from build123d import *

# Parameters (mm, degrees)
SKETCH1_W           = 76.2
SKETCH1_H           = 50.8
SKETCH1_R           = 3.175
SKETCH1_R_2         = 2.38125
BOSS_EXTRUDE1_DEPTH = 6.35


with BuildPart() as part:
    # Sketch1 → Boss-Extrude1 (new body)
    # profile 1 of 2: a face of its own
    with BuildSketch(Plane(origin=(0, 0, 0), x_dir=(1, 0, 0), z_dir=(0, 1, 0))):
        Rectangle(SKETCH1_W, SKETCH1_H)
        with Locations((25.4, 0)):
            Circle(SKETCH1_R, mode=Mode.SUBTRACT)
        with Locations(Location((-31.75, 0, 0), (0, 0, 270))):
            Circle(SKETCH1_R_2, mode=Mode.SUBTRACT)
    # profile 2 of 2: a face of its own
    with BuildSketch(Plane(origin=(0, 0, 0), x_dir=(1, 0, 0), z_dir=(0, 1, 0))):
        with Locations((25.4, 0)):
            Circle(SKETCH1_R)
    extrude(amount=BOSS_EXTRUDE1_DEPTH)


solid = part.part
Design review of the part built by this model. Coordinates are the model's own, in mm. Coordinates: 2 decimals unless noted, no trailing zeros. Order: outer loops, then holes, each group sorted by start corner. A loop starts at its lowest first (then second) coordinate and runs counter-clockwise, first axis right, second up.
Item 1: Take a section at B-B, the plane x = -31.75. Write out the cut boundary in (y, z), then the cut area to 3 significant figures.
Item 2: The part is to be moulded in two halves that separate along X. For faces 1 (the flat face through (-1, 0, 0)), 2 (the flat face through (-38.1, 3, 0)), 3 (the flat face through (38.1, 3, 0)), 4 (the cylindrical face through (-29.39, 3.13, -0.31)), say which applies: pulls with the +X half, pulls with the -X half, needs draft (parallel to the pull), parting line crosses it, or undercut.
Item 3: For pin 1 Ø1 at (x, z) = (8, -1) entering from -Y; pin 2 Ø3 at (x, z) = (-31.75, 0) entering from +Y, all flat-tipped, find the tip position at first contact; note any pin that passes through.
Item 4: Take a section at A-A, the plane z = 0. Write out the cut boundary in (x, y), then the cut area to 3 significant figures.
Item 5: For line 1 (X direction, y = 5, z = 0), list the stretches that pass through material, from the lowest coordinate up.
The answers:
1. outline: (0, -25.4) - (6.35, -25.4) - (6.35, -2.38) - (0, -2.38) - close; (0, 2.38) - (6.35, 2.38) - (6.35, 25.4) - (0, 25.4) - close
1. area: 292 mm2
2. face 1: needs draft
2. face 2: pulls with the -X half
2. face 3: pulls with the +X half
2. face 4: undercut
3. pin 1: stops at y = 0
3. pin 2: passes through
4. outline: (-38.1, 0) - (-34.13, 0) - (-34.13, 6.35) - (-38.1, 6.35) - close; (-29.37, 0) - (38.1, 0) - (38.1, 6.35) - (-29.37, 6.35) - close
4. area: 454 mm2
5. line 1: x = -38.1 to -34.13, -29.37 to 38.1
